The model under review builds one solid part; all positions refer to its coordinate system, in mm. A direction names the side the tool comes from. Round coordinates to 2 decimals unless told otherwise and drop trailing zeros. Loops run counter-clockwise (first coordinate to the right, second up) from the corner with the lowest first, then second, coordinate; pieces in that order, holes last. Notation, with made-up numbers: (-5, -40) -> (20, -40) arc R29 ccw to (20, -3) -> close; hole circle Ø10 at (-28, -13). An arc over 180 degrees is marked (long way). Use a Markdown table: item, result. Add a question column.
1) Consider section B-B on z = -34.5. Give the boundary of the cut face in (x, y).
2) For faces 1 (the flat face through (4, 17.5, -17)), 2 (the flat face through (4, 22, -20)), 3 (the flat face through (4, 1.15, -12)), 4 (the flat face through (1.972, 25.62, -41.106)), list the 3-axis set-ups (+Z, -Z, +X, -X, +Y, -Y) from which the entire face can be reached by the end or side of a thin tool; tool diameter is ignored.
3) Wall thickness on probe 1 along Y at (x, z) = (4, -15.75); probe 2 along Y at (x, z) = (2.25, -3.5); probe 3 along Z at (x, y) = (5.4, 23.25): over which ranges is each line inside the solid? List them lowest first.
4) Mouldability with a two-part tool opening along Y and no side actions: class faces 5 (the flat face through (2, 22, 0)), 6 (the cylindrical face through (4, 29, -49)), 7 (the flat face through (4, 0, -20)), 8 (the cylindrical face through (3.798, 23.037, -5.275)) as released by +Y, released by -Y, zero draft, split by the parting line, or undercut.
5) Consider section C-C on y = 28. Give the boundary of the cut face in (x, z), plus the area to 3 significant figures.
6) Insertion check: pin 1 (1.5 mm diameter, centred on x = 3.5, y = 22, fed in from +Z); pin 2 (1 mm diameter, centred on x = 1.5, y = 14, fed in from +Z); pin 3 (8 mm diameter, centred on y = 13, z = -19, fed in from +X); pin 4 (1.7 mm diameter, centred on x = 5, y = 5, fed in from -Z). Each pin has a flat end and moves straight along its axis. Give the tip position at first contact, or say it passes through.
7) Consider section A-A on x = 1. State how many separate pieces and enclosed holes the cut face has, plus the area to 3 significant figures.
from build123d import *

# Parameters (mm, degrees)
SKETCH1_R           = 1.55
BOSS_EXTRUDE1_DEPTH = 8
SKETCH4_R           = 1.55
CUT_EXTRUDE2_DEPTH  = 20
SKETCH5_W           = 2.6
SKETCH5_H           = 5.7
CUT_EXTRUDE3_DEPTH  = 60.371710435
FILLET2_R           = 1.5
FILLET3_R           = 5
FILLET4_R           = 10
CHAMFER1_SIZE       = 0.5
SKETCH6_R           = 2.5
SKETCH6_R_2         = 1.55
BOSS_EXTRUDE3_DEPTH = 0.75
CUT_EXTRUDE4_DEPTH  = 4


with BuildPart() as part:
    # Sketch1 → Boss-Extrude1 (new body)
    with BuildSketch(Plane(origin=(0, 0, 0), x_dir=(0, 0, -1), z_dir=(1, 0, 0))):
        Polygon((0, 0), (50, 0), (50, 31), (35, 31), (35, 25.5), (0, 25.5), (0, 17.5), (35, 17.5), (35, 8), (0, 8), align=None)
        with Locations((42.5, 23.25)):
            Circle(SKETCH1_R, mode=Mode.SUBTRACT)
    extrude(amount=BOSS_EXTRUDE1_DEPTH)

    # Sketch4 → Cut-Extrude2 (cut)
    with BuildSketch(Plane.XY):
        with Locations((4, 21.5)):
            Circle(SKETCH4_R)
        with Locations((4, 4)):
            Circle(SKETCH4_R)
    extrude(amount=-CUT_EXTRUDE2_DEPTH, mode=Mode.SUBTRACT)

    # Sketch5 → Cut-Extrude3 (cut, through all)
    with BuildSketch(Plane.ZY):
        with Locations((-12, 21.5)):
            Rectangle(SKETCH5_W, SKETCH5_H)
        with Locations((-12, 4)):
            Rectangle(SKETCH5_W, SKETCH5_H)
    extrude(amount=-CUT_EXTRUDE3_DEPTH, mode=Mode.SUBTRACT)

    # Fillet2
    fillet2_edges = [part.edges().sort_by_distance(p)[0] for p in [
        (4, 8, -35),
        (4, 17.5, -35),
        (4, 25.5, -35),
        (4, 31, -35),
    ]]
    fillet(fillet2_edges, radius=FILLET2_R)

    # Fillet3
    fillet3_edges = [part.edges().sort_by_distance(p)[0] for p in [
        (4, 31, -50),
    ]]
    fillet(fillet3_edges, radius=FILLET3_R)

    # Fillet4
    fillet4_edges = [part.edges().sort_by_distance(p)[0] for p in [
        (4, 0, -50),
    ]]
    fillet(fillet4_edges, radius=FILLET4_R)

    # Chamfer1
    chamfer1_edges = [part.edges().sort_by_distance(p)[0] for p in [
        (0, 21.5, 0),
        (0, 4, 0),
        (4, 8, 0),
        (4, 17.5, 0),
        (4, 25.5, 0),
        (4, 0, 0),
        (8, 21.5, 0),
        (8, 4, 0),
    ]]
    chamfer(chamfer1_edges, length=CHAMFER1_SIZE)

    # Sketch6 → Boss-Extrude3 (add)
    with BuildSketch(Plane(origin=(8, 0, 0), x_dir=(0, 0, -1), z_dir=(1, 0, 0))):
        with Locations((42.5, 23.25)):
            Circle(SKETCH6_R)
        with Locations((42.5, 23.25)):
            Circle(SKETCH6_R_2, mode=Mode.SUBTRACT)
    extrude(amount=BOSS_EXTRUDE3_DEPTH)

    # Sketch7 → Cut-Extrude4 (cut)
    with BuildSketch(Plane.ZY):
        Polygon((-39.750369343, 24.8375), (-42.5, 26.425), (-45.249630657, 24.8375), (-45.249630657, 21.6625), (-42.5, 20.075), (-39.750369343, 21.6625), align=None)
    extrude(amount=-CUT_EXTRUDE4_DEPTH, mode=Mode.SUBTRACT)


solid = part.part
Result set:
| question | item | result |
|---|---|---|
| 1 | outline | (0, 0) -> (8, 0) -> (8, 8.38) -> (0, 8.38) -> close; (0, 17.12) -> (8, 17.12) -> (8, 25.88) -> (0, 25.88) -> close |
| 2 | face 1 | +Z, +X, -X |
| 2 | face 2 | +Z |
| 2 | face 3 | +X, -X |
| 2 | face 4 | -X |
| 3 | probe 1 | 0 to 2.45, 5.55 to 8, 17.5 to 19.95, 23.05 to 25.5 |
| 3 | probe 2 | 0 to 8, 17.5 to 25.5 |
| 3 | probe 3 | -50 to -44.05, -40.95 to -13.3, -10.7 to 0 |
| 4 | face 5 | zero draft |
| 4 | face 6 | released by +Y |
| 4 | face 7 | released by -Y |
| 4 | face 8 | undercut |
| 5 | outline | (0, -49.58) -> (8, -49.58) -> (8, -35) -> (0, -35) -> close |
| 5 | area | 117 mm2 |
| 6 | pin 1 | z = -20 |
| 6 | pin 2 | z = -35 |
| 6 | pin 3 | through |
| 6 | pin 4 | z = -49.1 |
| 7 | separate pieces | 1 |
| 7 | enclosed holes | 3 |
| 7 | area | 943 mm2 |
